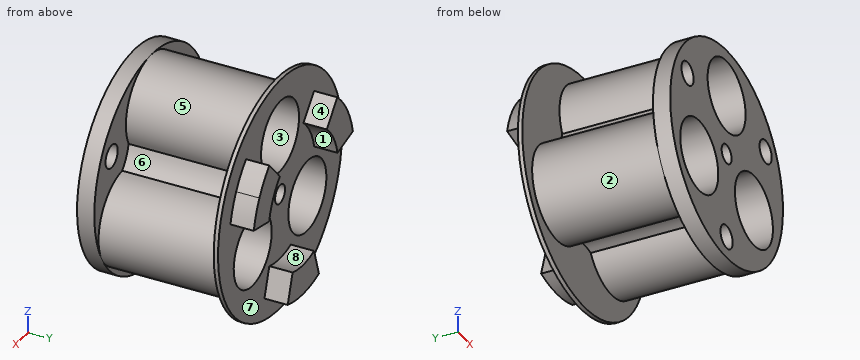
```python
from build123d import *

# Parameters (mm, degrees)
SKETCH1_R              = 27.5
SKETCH1_R_2            = 2.2
SKETCH1_R_3            = 8.425
BOSS_EXTRUDE1_DEPTH    = 34
BOSS_EXTRUDE2_DEPTH    = 5.4
CUT_EXTRUDE1_OUTLINE_R = 27.5
CUT_EXTRUDE1_DEPTH     = 29
SKETCH6_R              = 2.7
CUT_EXTRUDE2_DEPTH     = 5
SKETCH7_R              = 33.756466266
SKETCH7_R_2            = 27.5
SKETCH7_R_3            = 25
CUT_EXTRUDE6_DEPTH     = 4


# Read off the part's stored shape, not the designer's step: Cut-Extrude1
with BuildPart() as part:
    # Sketch1 → Boss-Extrude1 (new body)
    with BuildSketch(Plane(origin=(0, 0, 0), x_dir=(1, 0, 0), z_dir=(0, 1, 0))):
        with Locations(Location((0, 0, 0), (0, 0, 270))):
            Circle(SKETCH1_R)
        with Locations(Location((0, 0, 0), (0, 0, 270))):
            Circle(SKETCH1_R_2, mode=Mode.SUBTRACT)
        with Locations(Location((0, -14, 0), (0, 0, 270))):
            Circle(SKETCH1_R_3, mode=Mode.SUBTRACT)
        with Locations(Location((-12.124355653, 7, 0), (0, 0, 270))):
            Circle(SKETCH1_R_3, mode=Mode.SUBTRACT)
        with Locations(Location((12.124355653, 7, 0), (0, 0, 270))):
            Circle(SKETCH1_R_3, mode=Mode.SUBTRACT)
    extrude(amount=BOSS_EXTRUDE1_DEPTH)

    # Sketch4 → Boss-Extrude2 (add)
    with BuildSketch(Plane(origin=(0, 34, 0), x_dir=(1, 0, 0), z_dir=(0, 1, 0))):
        with BuildLine():
            ThreePointArc((-22.000122827, -4.716417665), (-19.485571585, -11.25), (-15.084598927, -16.694456422))
            Line((-15.084598927, -16.694456422), (-10.391612594, -11.500625535))
            ThreePointArc((-10.391612594, -11.500625535), (-13.423393759, -7.75), (-15.15564017, -3.249087725))
            Line((-15.15564017, -3.249087725), (-22.000122827, -4.716417665))
        make_face()
        with BuildLine():
            Line((4.764027576, 14.74971326), (6.9155239, 21.410874087))
            ThreePointArc((6.9155239, 21.410874087), (0, 22.5), (-6.9155239, 21.410874087))
            Line((-6.9155239, 21.410874087), (-4.764027576, 14.74971326))
            ThreePointArc((-4.764027576, 14.74971326), (0, 15.5), (4.764027576, 14.74971326))
        make_face()
        with BuildLine():
            Line((19.485571585, -11.25), (13.423393759, -7.75))
            ThreePointArc((13.423393759, -7.75), (12.054270192, -9.743950438), (10.391612594, -11.500625535))
            Line((10.391612594, -11.500625535), (15.084598927, -16.694456422))
            ThreePointArc((15.084598927, -16.694456422), (17.49813415, -14.144444184), (19.485571585, -11.25))
        make_face()
        with BuildLine():
            ThreePointArc((15.15564017, -3.249087725), (14.465643708, -5.567328992), (13.423393759, -7.75))
            Line((13.423393759, -7.75), (19.485571585, -11.25))
            ThreePointArc((19.485571585, -11.25), (20.998515061, -8.081606601), (22.000122827, -4.716417665))
            Line((22.000122827, -4.716417665), (15.15564017, -3.249087725))
        make_face()
    extrude(amount=BOSS_EXTRUDE2_DEPTH)

    # Cut-Extrude1 outline → Cut-Extrude1 (cut)
    with BuildSketch(Plane(origin=(0, 4, 0), x_dir=(1, 0, 0), z_dir=(0, 1, 0))):
        Circle(CUT_EXTRUDE1_OUTLINE_R)
        with BuildLine():
            ThreePointArc((12.609360996, -3.989302517), (10.825317547, -6.25), (9.759517821, -8.925375689))
            ThreePointArc((9.759517821, -8.925375689), (0, -25), (-9.759517821, -8.925375689))
            ThreePointArc((-9.759517821, -8.925375689), (-10.825317547, -6.25), (-12.609360996, -3.989302517))
            ThreePointArc((-12.609360996, -3.989302517), (-21.650635095, 12.5), (-2.849843175, 12.914678207))
            ThreePointArc((-2.849843175, 12.914678207), (0, 12.5), (2.849843175, 12.914678207))
            ThreePointArc((2.849843175, 12.914678207), (21.650635095, 12.5), (12.609360996, -3.989302517))
        make_face(mode=Mode.SUBTRACT)
    extrude(amount=CUT_EXTRUDE1_DEPTH, mode=Mode.SUBTRACT)

    # Sketch6 → Cut-Extrude2 (cut)
    with BuildSketch(Plane.XZ):
        with Locations(Location((0, -20, 0), (0, 0, 270))):
            Circle(SKETCH6_R)
        with Locations(Location((-17.320508076, 10, 0), (0, 0, 270))):
            Circle(SKETCH6_R)
        with Locations(Location((17.320508076, 10, 0), (0, 0, 270))):
            Circle(SKETCH6_R)
    extrude(amount=-CUT_EXTRUDE2_DEPTH, mode=Mode.SUBTRACT)

    # Sketch7 → Cut-Extrude6 (cut)
    # profile 1 of 2: a face of its own
    with BuildSketch(Plane.XZ):
        Circle(SKETCH7_R)
        with Locations(Location((0, 0, 0), (0, 0, 90))):
            Circle(SKETCH7_R_2, mode=Mode.SUBTRACT)
    # profile 2 of 2: a face of its own
    with BuildSketch(Plane.XZ):
        with Locations(Location((0, 0, 0), (0, 0, 90))):
            Circle(SKETCH7_R_2)
        with Locations(Location((0, 0, 0), (0, 0, 270))):
            Circle(SKETCH7_R_3, mode=Mode.SUBTRACT)
    extrude(amount=-CUT_EXTRUDE6_DEPTH, mode=Mode.SUBTRACT)


solid = part.part
```
Model file for the job. Use its own axes, mm. Face numbers are marked on the shaded views. A direction names the side the tool comes from. Give positions to 0.01 mm unless a question says otherwise; leave off trailing zeros. Write each loop counter-clockwise with the first axis right and the second up, starting at its lowest first coordinate (ties: lowest second). Pieces come first, ordered by that corner, then holes. Notation, with made-up numbers: M -15,-1 L 1,-1 A13 ccw 1,21 Z; hole C 7.25,23.5 d6. An arc over 180 degrees is marked long. Use a Markdown table: item, result.
1) Cut at B-B (y = 2.5). Give the number of separate pieces and of enclosed holes in the cut face, and give its area (3 significant figures).
Responses:
| item | result |
|---|---|
| separate pieces | 1 |
| enclosed holes | 7 |
| area | 1,210 mm2 |
2) Pull direction Z, two halves, no side cores. Call the marked faces 1, 2, 3 and 4: +Z half, -Z half, draft (parallel to the pull), parting line (faces both ways), or undercut.
Responses:
| item | result |
|---|---|
| face 1 | -Z half |
| face 2 | parting line |
| face 3 | undercut |
| face 4 | +Z half |
3) Pin check, flat tips, straight feed: pin 1 (8 mm diameter, centred on y = 32, z = 14.5, fed in from +X); pin 2 (1 mm diameter, centred on x = -7, y = 22, fed in from -Z); pin 3 (12 mm diameter, centred on x = -16, y = 20.5, fed in from +Z). Stop position of each tip, or through.
Responses:
| item | result |
|---|---|
| pin 1 | stops at x = 25.36 |
| pin 2 | stops at z = -16.98 |
| pin 3 | stops at z = 18.58 |
4) Tool access for the marked faces 5, 6, 7 and 8: list every direction of +Z, -Z, +X, -X, +Y, -Y with a clear straight run to the whole face (end or side of a thin tool).
Responses:
| item | result |
|---|---|
| face 5 | none |
| face 6 | +X |
| face 7 | +Y |
| face 8 | +Z, +Y |
5) Cut at A-A (z = -20). List the corners of the cut face in (x, y).
Responses:
| item | result |
|---|---|
| outline | M -18.87,33 L 18.87,33 L 18.87,34 L 6.46,34 L 6.46,39.4 L -6.46,39.4 L -6.46,34 L -18.87,34 Z; M -15,0 L -2.7,0 L -2.7,4 L -15,4 Z; M 2.7,0 L 15,0 L 15,4 L 2.7,4 Z |
6) Cut at D-D (y = 32). List the corners of the cut face in (x, z) (3 decimals), and give its area (3 significant figures).
Responses:
| item | result |
|---|---|
| outline | M -12.609,3.989 A11 ccw long -2.85,-12.915 A10 cw 2.85,-12.915 A11 ccw long 12.609,3.989 A10 cw 9.76,8.925 A11 ccw long -9.76,8.925 A10 cw Z; hole C -12.124,-7 d16.85; hole C 0,14 d16.85; hole C 0,0 d4.4; hole C 12.124,-7 d16.85 |
| area | 576 mm2 |
7) Drill centre lines: line 1 (X direction, y = 26, z = -7); line 2 (Y direction, x = -23, z = 0.5); line 3 (Z direction, x = -6, y = 13.5). Where is each one in solid material? Low to high. Write a range as from..to.
Responses:
| item | result |
|---|---|
| line 1 | x = -23.12..-20.55, -3.7..3.7, 20.55..23.12 |
| line 2 | y = 0..4, 33..34 |
| line 3 | z = -16.14..-12.79, -1.21..8.09, 19.91..23.22 |
